```python
from build123d import *

# Parameters (mm, degrees)
ESBO_O1_W                = 120
ESBO_O1_H                = 80
RESSALTO_EXTRUS_O2_DEPTH = 2
ESBO_O2_W                = 120
ESBO_O2_H                = 80
ESBO_O2_W_2              = 116
ESBO_O2_H_2              = 76
EXTRUS_O_FINA1_DEPTH     = 13
CORTE_EXTRUS_O1_DEPTH    = 2


with BuildPart() as part:
    # Esboço1 → Ressalto-extrusão2 (new body)
    with BuildSketch(Plane(origin=(0, 0, 0), x_dir=(1, 0, 0), z_dir=(0, 1, 0))):
        Rectangle(ESBO_O1_W, ESBO_O1_H)
    extrude(amount=RESSALTO_EXTRUS_O2_DEPTH)

    # Esboço2 → Extrusão-Fina1 (add)
    with BuildSketch(Plane(origin=(0, 2, 0), x_dir=(1, 0, 0), z_dir=(0, 1, 0))):
        Rectangle(ESBO_O2_W, ESBO_O2_H)
        Rectangle(ESBO_O2_W_2, ESBO_O2_H_2, mode=Mode.SUBTRACT)
    extrude(amount=EXTRUS_O_FINA1_DEPTH)

    # Esboço3 → Corte-extrusão1 (cut)
    with BuildSketch(Plane.XY.offset(40)):
        with BuildLine():
            Line((-15, 10), (15, 10))
            ThreePointArc((15, 10), (17.5, 7.5), (15, 5))
            Line((15, 5), (-15, 5))
            ThreePointArc((-15, 5), (-17.5, 7.5), (-15, 10))
        make_face()
    extrude(amount=-CORTE_EXTRUS_O1_DEPTH, mode=Mode.SUBTRACT)


solid = part.part
```
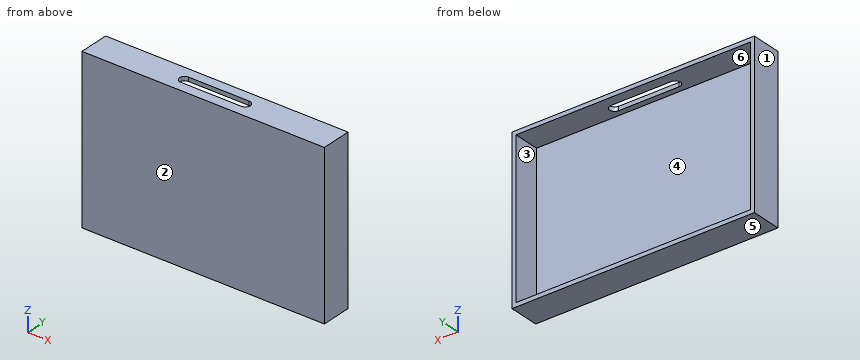
Source: CAD feature listing. Evaluate the final solid. Frame: model axes, mm. Face numbers are marked on the shaded views. A direction names the side the tool comes from. Coordinates: 2 decimals unless noted, no trailing zeros. Write each loop counter-clockwise with the first axis right and the second up, starting at its lowest first coordinate (ties: lowest second). Pieces come first, ordered by that corner, then holes. Notation, with made-up numbers: (-10, 1.25) -> (11, 1.25) arc R25 cw to (11, 40.25) -> close; hole circle Ø10 at (11.5, 37). An arc over 180 degrees is marked (long way). Return JSON: item names as keys, results as strings. Group by question number.
1) Section query C-C, the plane z = 19. Return loops of the section in (x, y).
2) Mould query, pull axis X, two halves, no side actions, for the marked faces 1, 2, 3 and 4. Classes: +X half, -X half, draft (parallel to the pull), parting line (faces both ways), or undercut.
3) Ray query, line 1 along X through (y, z) = (4.75, -32.5); line 2 along Z through (x, y) = (3, 3.5); line 3 along Y through (x, z) = (11.5, -2.5). Return the intervals inside material, ascending.
4) Contact query for a flat-ended pin moving along its axis: P1, Ø10, axis at x = 6.5, z = -3.5, coming from the +Y side. Output: stop coordinate, or through.
5) Set-up query: the marked faces 5 and 6. Return all of +Z, -Z, +X, -X, +Y, -Y with unobstructed straight access to the full face (end or side cutting, diameter ignored); none if empty.
6) Section query B-B, the plane y = 13.5. Return loops of the section in (x, z), plus the area to 3 significant figures.
7) Section query A-A, the plane x = -4.5. Return loops of the section in (y, z).
8) Section query D-D, the plane x = 45. Return loops of the section in (y, z), plus the area to 3 significant figures.
From the geometry:
{
 "1": {"outline": "(-60, 0) -> (60, 0) -> (60, 15) -> (58, 15) -> (58, 2) -> (-58, 2) -> (-58, 15) -> (-60, 15) -> close"},
 "2": {"face 1": "-X half", "face 2": "draft", "face 3": "undercut", "face 4": "undercut"},
 "3": {"line 1": "-60 to -58, 58 to 60", "line 2": "-40 to -38, 38 to 40", "line 3": "0 to 2"},
 "4": {"P1": "y = 2"},
 "5": {"face 5": "-Z, +X, -X, +Y, -Y", "face 6": "+Y"},
 "6": {"outline": "(-60, -40) -> (60, -40) -> (60, 40) -> (-60, 40) -> close; hole (-58, -38) -> (58, -38) -> (58, 38) -> (-58, 38) -> close", "area": "784 mm²"},
 "7": {"outline": "(0, -40) -> (15, -40) -> (15, -38) -> (2, -38) -> (2, 38) -> (5, 38) -> (5, 40) -> (0, 40) -> close; (10, 38) -> (15, 38) -> (15, 40) -> (10, 40) -> close"},
 "8": {"outline": "(0, -40) -> (15, -40) -> (15, -38) -> (2, -38) -> (2, 38) -> (15, 38) -> (15, 40) -> (0, 40) -> close", "area": "212 mm²"}
}
